Verification items for the finished model (mm, model axes). Round coordinates to 2 decimals unless told otherwise and drop trailing zeros. Write each loop counter-clockwise with the first axis right and the second up, starting at its lowest first coordinate (ties: lowest second). Pieces come first, ordered by that corner, then holes. Notation, with made-up numbers: M -21.75,71.25 L 15.25,71.25 A30 ccw 15.25,102.25 Z; hole C 32,8.25 d1. An arc over 180 degrees is marked long. Answer in a Markdown table with one row per item. Add a question column.
1. Go/stop test with a flat-tipped pin: pin 1 Ø11.5 at (x, y) = (0, -18) entering from -Z. Record where the tip stops, or that it passes through.
2. Sectioned sample at A-A on x = 14. Record the cut outline in (y, z), plus the area to 3 significant figures.
3. Draft check along Y on faces 1 (the flat face through (-5, 25, -2)), 2 (the flat face through (-1, 0, -5)), 3 (the cylindrical face through (-1.08, -22.88, -2.46)), 4 (the cylindrical face through (13, 0, -2)). Enter one of: pulls with the +Y half, pulls with the -Y half, needs draft (parallel to the pull), parting line crosses it, or undercut.
4. Sectioned sample at D-D on z = -0.85. Record the cut outline in (x, y).
5. Sectioned sample at B-B on y = 0. Record the cut outline in (x, z), plus the area to 3 significant figures.
6. Sectioned sample at C-C on x = 0. Record the cut outline in (y, z), plus the area to 3 significant figures.
7. Material ranges on probe 1 along Y at (x, z) = (0, -3.3); probe 2 along X at (y, z) = (-4.5, -2.9); probe 3 along X at (y, z) = (-2, -1.05), recorded low to high.
```python
from build123d import *

# Parameters (mm, degrees)
SKETCH2_W           = 80
SKETCH2_H           = 50
BOSS_EXTRUDE1_DEPTH = 5
SKETCH3_R           = 5
CUT_EXTRUDE1_DEPTH  = 5
FILLET1_R           = 10


with BuildPart() as part:
    # Sketch2 → Boss-Extrude1 (new body)
    with BuildSketch(Plane.XY):
        Rectangle(SKETCH2_W, SKETCH2_H)
    extrude(amount=-BOSS_EXTRUDE1_DEPTH)

    # Sketch3 → Cut-Extrude1 (cut)
    with BuildSketch(Plane.XY):
        with Locations((-18, 0)):
            Circle(SKETCH3_R)
        with Locations((0, 18)):
            Circle(SKETCH3_R)
        with Locations((18, 0)):
            Circle(SKETCH3_R)
        with Locations((0, -18)):
            Circle(SKETCH3_R)
    extrude(amount=-CUT_EXTRUDE1_DEPTH, mode=Mode.SUBTRACT)

    # Fillet1
    fillet1_edges = [part.edges().sort_by_distance(p)[0] for p in [
        (40, 25, -2.5),
    ]]
    fillet(fillet1_edges, radius=FILLET1_R)


solid = part.part
```
Geometry check:
| question | item | result |
|---|---|---|
| 1 | pin 1 | stops at z = -5 |
| 2 | outline | M -25,-5 L -3,-5 L -3,0 L -25,0 Z; M 3,-5 L 25,-5 L 25,0 L 3,0 Z |
| 2 | area | 220 mm2 |
| 3 | face 1 | pulls with the +Y half |
| 3 | face 2 | needs draft |
| 3 | face 3 | undercut |
| 3 | face 4 | undercut |
| 4 | outline | M -40,-25 L 40,-25 L 40,15 A10 ccw 30,25 L -40,25 Z; hole C -18,0 d10; hole C 0,-18 d10; hole C 0,18 d10; hole C 18,0 d10 |
| 5 | outline | M -40,-5 L -23,-5 L -23,0 L -40,0 Z; M -13,-5 L 13,-5 L 13,0 L -13,0 Z; M 23,-5 L 40,-5 L 40,0 L 23,0 Z |
| 5 | area | 300 mm2 |
| 6 | outline | M -25,-5 L -23,-5 L -23,0 L -25,0 Z; M -13,-5 L 13,-5 L 13,0 L -13,0 Z; M 23,-5 L 25,-5 L 25,0 L 23,0 Z |
| 6 | area | 150 mm2 |
| 7 | probe 1 | y = -25 to -23, -13 to 13, 23 to 25 |
| 7 | probe 2 | x = -40 to -20.18, -15.82 to 15.82, 20.18 to 40 |
| 7 | probe 3 | x = -40 to -22.58, -13.42 to 13.42, 22.58 to 40 |
